Read the model definition and answer for the solid it produces. Units are mm, in the model's axes. A direction names the side the tool comes from. Give positions to 0.01 mm unless a question says otherwise; leave off trailing zeros. Order: outer loops, then holes, each group sorted by start corner. A loop starts at its lowest first (then second) coordinate and runs counter-clockwise, first axis right, second up. Notation, with made-up numbers: (10.5, 3.25) - (54.5, 3.25) arc R21 cw to (54.5, 25.25) - close; hole circle Ø5 at (-24.5, -8). An arc over 180 degrees is marked (long way). Write each question's results on one line, items separated by ' | '.
from build123d import *

# Parameters (mm, degrees)
F0_R      = 88.9
F1_DEPTH  = 873.125
F1_FACE_R = 88.9
F3_R      = 69.85
F5_R      = 50.8
F6_DEPTH  = 66.802
F7_SIZE   = 1.524


with BuildPart() as f1:
    # F0 (on Right) → F1 (new body, symmetric)
    with BuildSketch(Plane.YZ):
        Circle(F0_R)
    extrude(amount=F1_DEPTH, both=True)

    # F1_face (on face) → F4 section 0
    with BuildSketch(Plane.YZ.offset(873.125)):
        Circle(F1_FACE_R)
    # F3 (on offset) → F4 section 1
    with BuildSketch(Plane.YZ.offset(1101.725)):
        Circle(F3_R)
    loft()

    # F5 (on face) → F6 (join)
    with BuildSketch(Plane.YZ.offset(1101.725)):
        Circle(F5_R)
    extrude(amount=F6_DEPTH)

    # F7
    f7_edges = [f1.edges().sort_by_distance(p)[0] for p in [
        (1168.527, -50.8, 0),
    ]]
    chamfer(f7_edges, length=F7_SIZE)

    # F8: F1 across plane


with BuildPart() as f1_1:
    add(f1.part)
    add(f1.part.mirror(Plane.YZ))


solid = f1_1.part
(1) For faces 1 (the face through (1101.725, 5, -51)), 2 (the face through (-1101.725, 5, -51)), 3 (the face through (-1168.527, -1, 1)), determine the directions among +Z, -Z, +X, -X, +Y, -Y from which every point of the face is accessible in a straight line to the end or side of a thin tool.
Conclusion:
face 1: +X | face 2: -X | face 3: +Z, -Z, -X, +Y, -Y
(2) Section A-A (y = 0) is taken. Give the vertices of the cut face in (x, z) (3 decimals).
Conclusion:
outline: (-1168.527, -49.276) - (-1167.003, -50.8) - (-1101.725, -50.8) - (-1101.725, -69.85) - (-873.125, -88.9) - (873.125, -88.9) - (1101.725, -69.85) - (1101.725, -50.8) - (1167.003, -50.8) - (1168.527, -49.276) - (1168.527, 49.276) - (1167.003, 50.8) - (1101.725, 50.8) - (1101.725, 69.85) - (873.125, 88.9) - (-873.125, 88.9) - (-1101.725, 69.85) - (-1101.725, 50.8) - (-1167.003, 50.8) - (-1168.527, 49.276) - close
(3) Section B-B (x = 411) is taken. Give the vertices of the cut face in (y, z).
Conclusion:
outline: circle Ø177.8 at (0, 0)
(4) Consider probe 1 along Y at (x, z) = (-1048, 25); probe 2 along X at (y, z) = (-55.5, -38) (3 decimals); probe 3 along Y at (x, z) = (554, -54.5). Determine where each line is inside the solid, lowest interval first. Write a range as [from, to].
Conclusion:
probe 1: [-70, 70] | probe 2: [-1101.725, 1101.725] | probe 3: [-70.24, 70.24]
(5) Each of these flat-tipped pins is pushed along its axis until it touches: pin 1 (4 mm diameter, centred on x = 744.5, y = -67, fed in from +Z); pin 2 (12 mm diameter, centred on x = 577, y = 36.5, fed in from -Z); pin 3 (8 mm diameter, centred on y = -62, z = -38, fed in from +X) (3 decimals). Where does it stop, or does it pass through?
Conclusion:
pin 1: z = 60.65 | pin 2: z = -83.5 | pin 3: x = 1101.725
